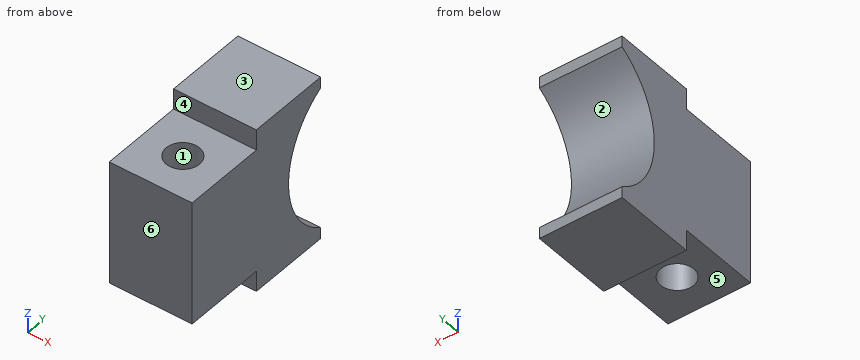
from build123d import *

# Parameters (mm, degrees)
SKETCH1_W               = 12.7
SKETCH1_H               = 25.4
BOSS_EXTRUDE1_DEPTH     = 25.4
SKETCH2_OUTSIDE_W       = 35.02
SKETCH2_OUTSIDE_H       = 35.02
CUT_EXTRUDE1_DEPTH      = 13.7
F_1_4_20_TAPPED_HOLE2_D = 5.1054


with BuildPart() as part:
    # Sketch1 → Boss-Extrude1 (new body)
    with BuildSketch(Plane.XY):
        Rectangle(SKETCH1_W, SKETCH1_H)
    extrude(amount=BOSS_EXTRUDE1_DEPTH)

    # Sketch2 outside → Cut-Extrude1 (cut, through all)
    with BuildSketch(Plane.ZY.offset(6.35)):
        with Locations((12.7, 0)):
            Rectangle(SKETCH2_OUTSIDE_W, SKETCH2_OUTSIDE_H)
        with BuildLine():
            Line((23.698522628, 12.7), (25.4, 12.7))
            Line((25.4, 12.7), (25.4, 0))
            Line((25.4, 0), (22.225, 0))
            Line((22.225, 0), (22.225, -12.7))
            Line((22.225, -12.7), (3.175, -12.7))
            Line((3.175, -12.7), (3.175, 0))
            Line((3.175, 0), (0, 0))
            Line((0, 0), (0, 12.7))
            Line((0, 12.7), (1.701477372, 12.7))
            ThreePointArc((1.701477372, 12.7), (12.7, 6.35), (23.698522628, 12.7))
        make_face(mode=Mode.SUBTRACT)
    extrude(amount=-CUT_EXTRUDE1_DEPTH, mode=Mode.SUBTRACT)

    # 1/4-20 Tapped Hole2 (through all)
    with Locations(Plane(origin=(0, -6.35, 3.175), x_dir=(0, -1, 0), z_dir=(0, 0, -1))):
        with Locations((0, 0)):
            Hole(F_1_4_20_TAPPED_HOLE2_D / 2)


solid = part.part
Work out the finished part from the listing and answer in its coordinate system (mm). Face numbers are marked on the shaded views. A direction names the side the tool comes from. Give positions to 0.01 mm unless a question says otherwise; leave off trailing zeros. Loops run counter-clockwise (first coordinate to the right, second up) from the corner with the lowest first, then second, coordinate; pieces in that order, holes last. Notation, with made-up numbers: (72.25, -18.75) -> (128.25, -18.75) arc R33 cw to (128.25, 9.25) -> close; hole circle Ø9 at (-8.75, 29). An arc over 180 degrees is marked (long way). Use a Markdown table: item, result. Add a question column.
1) The part is cut by section B-B, the plane y = -6.35. Determine the outline of the cut face in (x, z) (3 decimals).
2) The part is cut by section A-A, the plane x = 0. Determine the outline of the cut face in (y, z) (3 decimals), plus the area to 3 significant figures.
3) For a pull along Y with two mould halves and no side action, classify the marked faces 1, 2 and 3 as +Y half, -Y half, draft (parallel to the pull), parting line (faces both ways), or undercut.
4) Each of these flat-tipped pins is pushed along its axis until it touches: P1, Ø5, axis at x = 4, z = 18, coming from the +Y side; P2, Ø1, axis at x = -2.5, z = 2.5, coming from the -Y side; P3, Ø6.5, axis at x = -0.5, y = -8, coming from the -Z side (3 decimals). Where does it stop, or does it pass through?
5) The part is cut by section D-D, the plane x = 5. Determine the outline of the cut face in (y, z) (3 decimals).
6) Which of the six approach directions +Z, -Z, +X, -X, +Y, -Y give full straight-line access (tool end or side, diameter ignored) to the marked faces 4, 5 and 6?
7) Consider line 1 along X through (y, z) = (-6.35, 7.5); line 2 along Z through (x, y) = (-4, -10.5) (3 decimals); line 3 along Z through (x, y) = (-3.5, 10). Determine where each line is inside the solid, lowest interval first.
8) The part is cut by section C-C, the plane z = 7.5. Determine the outline of the cut face in (x, y).
Reported:
| question | item | result |
|---|---|---|
| 1 | outline | (-6.35, 3.175) -> (-2.553, 3.175) -> (-2.553, 22.225) -> (-6.35, 22.225) -> close; (2.553, 3.175) -> (6.35, 3.175) -> (6.35, 22.225) -> (2.553, 22.225) -> close |
| 2 | outline | (-12.7, 3.175) -> (-8.903, 3.175) -> (-8.903, 22.225) -> (-12.7, 22.225) -> close; (-3.797, 3.175) -> (0, 3.175) -> (0, 0) -> (12.7, 0) -> (12.7, 1.701) arc R12.7 cw to (12.7, 23.699) -> (12.7, 25.4) -> (0, 25.4) -> (0, 22.225) -> (-3.797, 22.225) -> close |
| 2 | area | 368 mm^2 |
| 3 | face 1 | undercut |
| 3 | face 2 | +Y half |
| 3 | face 3 | draft |
| 4 | P1 | stops at y = 9.03 |
| 4 | P2 | stops at y = 0 |
| 4 | P3 | stops at z = 3.175 |
| 5 | outline | (-12.7, 3.175) -> (0, 3.175) -> (0, 0) -> (12.7, 0) -> (12.7, 1.701) arc R12.7 cw to (12.7, 23.699) -> (12.7, 25.4) -> (0, 25.4) -> (0, 22.225) -> (-12.7, 22.225) -> close |
| 6 | face 4 | +Z, +X, -X, -Y |
| 6 | face 5 | -Z, +X, -X, -Y |
| 6 | face 6 | +Z, -Z, +X, -X, -Y |
| 7 | line 1 | x = -6.35 to -2.55, 2.55 to 6.35 |
| 7 | line 2 | z = 3.175 to 22.225 |
| 7 | line 3 | z = 0 to 3.79, 21.61 to 25.4 |
| 8 | outline | (-6.35, -12.7) -> (6.35, -12.7) -> (6.35, 7.46) -> (-6.35, 7.46) -> close; hole circle Ø5.11 at (0, -6.35) |
